Could you check a few things on this model? Use its own coordinates, in mm. Give positions to 0.01 mm unless a question says otherwise; leave off trailing zeros. Order: outer loops, then holes, each group sorted by start corner. A loop starts at its lowest first (then second) coordinate and runs counter-clockwise, first axis right, second up. Notation, with made-up numbers: M 75.5,46.5 L 88.5,46.5 A23 ccw 88.5,60.5 Z; hole C 49,40.25 d6. An arc over 180 degrees is marked long. Return JSON: item names as keys, results as strings. Group by question number.
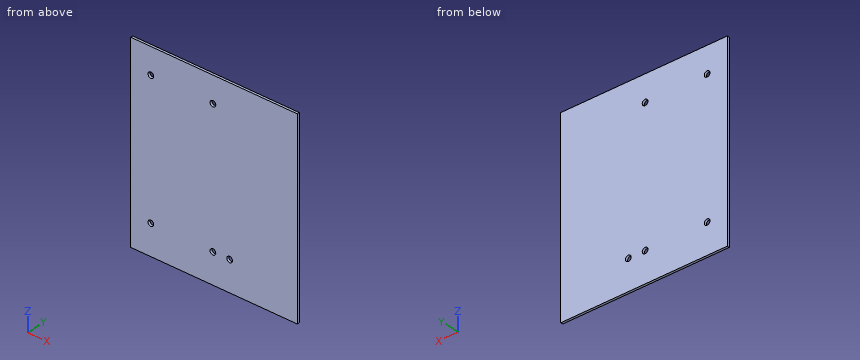
```python
from build123d import *

# Parameters (mm, degrees)
F0_W     = 254
F0_H     = 289.306
F1_DEPTH = 3.556
F2_R     = 4.375282
F3_DEPTH = 25.4
F4_DEPTH = 25.4


with BuildPart() as f1:
    # F0 (on Front) → F1 (new body)
    with BuildSketch(Plane.XZ):
        with Locations((67.888133, 103.692655)):
            Rectangle(F0_W, F0_H)
    extrude(amount=F1_DEPTH)

    # F2 (on face) → F3 (cut)
    with BuildSketch(Plane.XZ.offset(3.556)):
        with Locations((-28.39225, 4.948523)):
            Circle(F2_R)
    extrude(amount=-F3_DEPTH, mode=Mode.SUBTRACT)

    # F2 (on face) → F4 (cut)
    with BuildSketch(Plane.XZ.offset(3.556)):
        with Locations((-28.39225, 4.948523)):
            Circle(F2_R)
        with Locations((-28.39225, 208.903685)):
            Circle(F2_R)
        with Locations((66.210382, 4.948523)):
            Circle(F2_R)
        with Locations((66.210382, 208.903685)):
            Circle(F2_R)
        with Locations((91.772243, 4.948523)):
            Circle(F2_R)
    extrude(amount=-F4_DEPTH, mode=Mode.SUBTRACT)


solid = f1.part
```
1. Imagine slicing it at A-A, the plane x = 93. Please give me the cut outline in (y, z), plus the area to 3 significant figures.
2. For pin 1 (5.5 mm diameter, centred on x = -28.39, z = 208.9, fed in from +Y), with a flat end and sliding along its axis, tell me the tip position at first contact or that it passes through.
3. I need wall thicknesses on L1, parallel to Z at x = 66.5, y = -0.75; L2, parallel to X at y = -1.4, z = 212. Which ranges of each line are inside material? Lowest first, please. Write a range as from..to.
Values:
{
 "1": {"outline": "M -3.56,-40.96 L 0,-40.96 L 0,0.75 L -3.56,0.75 Z; M -3.56,9.15 L 0,9.15 L 0,248.35 L -3.56,248.35 Z", "area": "999 mm²"},
 "2": {"pin 1": "passes through"},
 "3": {"L1": "z = -40.96..0.58, 9.31..204.54, 213.27..248.35", "L2": "x = -59.11..-31.48, -25.3..63.12, 69.3..194.89"}
}
